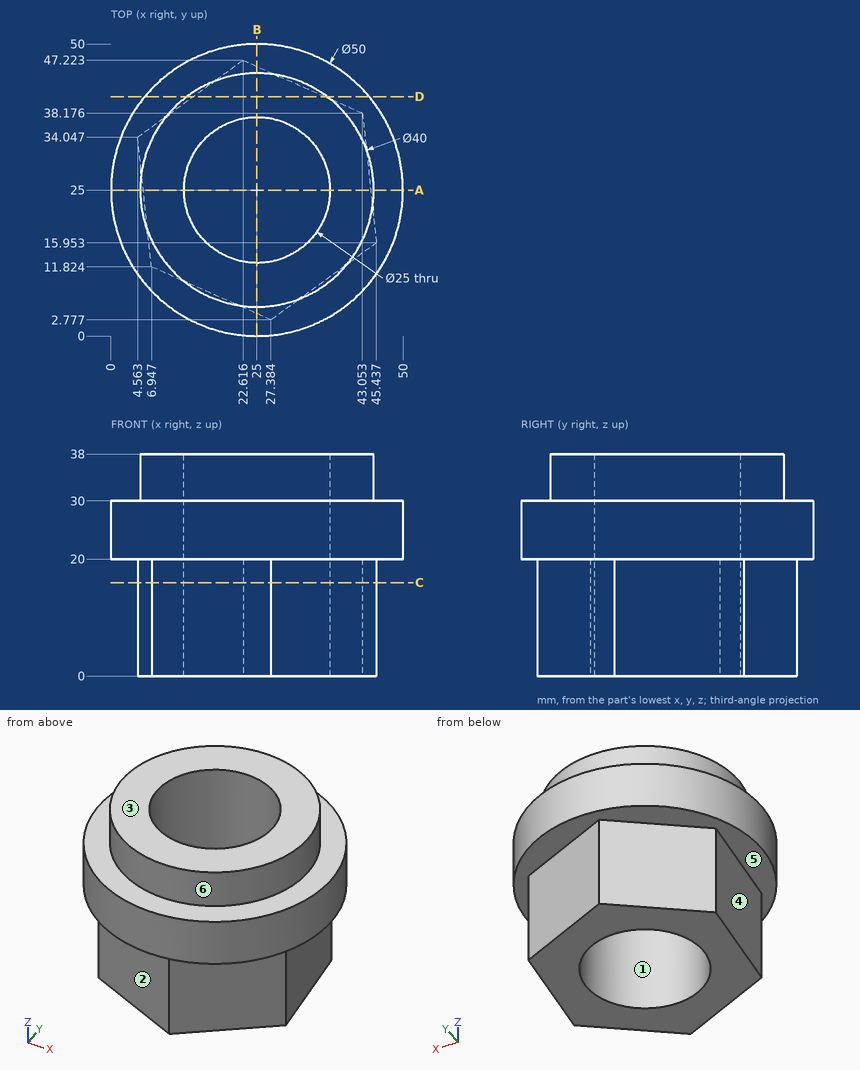
Job drawing, mm, ordinate dimensions from the low corner. One solid piece. A direction names the side the tool comes from. Coordinates: 2 decimals unless noted, no trailing zeros. Order: outer loops, then holes, each group sorted by start corner. A loop starts at its lowest first (then second) coordinate and runs counter-clockwise, first axis right, second up. Notation, with made-up numbers: M 80.25,82 L 129.25,82 A20 ccw 129.25,108 Z; hole C 88,-15.5 d6. An arc over 180 degrees is marked long. Return JSON: item names as keys, results as strings.
1. Pull direction X, two halves, no side cores. Call the marked faces 1, 2 and 3: +X half, -X half, draft (parallel to the pull), parting line (faces both ways), or undercut.
Ans:
{"face 1": "undercut", "face 2": "-X half", "face 3": "draft"}
2. Tool access for the marked faces 4, 5 and 6: list every direction of +Z, -Z, +X, -X, +Y, -Y with a clear straight run to the whole face (end or side of a thin tool).
Ans:
{"face 4": "-Z, -X, -Y", "face 5": "-Z", "face 6": "+Z"}
3. Saw through at A-A (y = 25). Give the cut face in (x, z).
Ans:
{"outline": "M 0,20 L 5.53,20 L 5.53,0 L 12.5,0 L 12.5,38 L 5,38 L 5,30 L 0,30 Z; M 37.5,0 L 44.47,0 L 44.47,20 L 50,20 L 50,30 L 45,30 L 45,38 L 37.5,38 Z"}
4. Saw through at B-B (x = 25). Give the cut face in (y, z).
Ans:
{"outline": "M 0,20 L 3.83,20 L 3.83,0 L 12.5,0 L 12.5,38 L 5,38 L 5,30 L 0,30 Z; M 37.5,0 L 46.17,0 L 46.17,20 L 50,20 L 50,30 L 45,30 L 45,38 L 37.5,38 Z"}
5. Flat gauge pins, fed straight in: pin 1 (10 mm diameter, centred on y = 11.5, z = 6.5, fed in from -X) (1 decimal); pin 2 (25 mm diameter, centred on x = 37, y = 18.5, fed in from -Z); pin 3 (5 mm diameter, centred on y = 34, z = 28.5, fed in from +X); pin 4 (2 mm diameter, centred on y = 11, z = 29, fed in from +X) (1 decimal). Where does each tip first touch, or does it go through?
Ans:
{"pin 1": "x = 6.4", "pin 2": "z = 0", "pin 3": "x = 49.14", "pin 4": "x = 46.4"}
6. Drill centre lines: probe 1 along Y at (x, z) = (25, 23.5); probe 2 along Y at (x, z) = (33.5, 25) (1 decimal); probe 3 along Z at (x, y) = (9.5, 42.5). Where is each one in solid material? Low to high.
Ans:
{"probe 1": "0 to 12.5, 37.5 to 50", "probe 2": "1.5 to 15.8, 34.2 to 48.5", "probe 3": "20 to 30"}
7. Saw through at D-D (y = 41). Give the cut face in (x, z), and give its area (3 significant figures).
Ans:
{"outline": "M 5.79,20 L 14.09,20 L 14.09,0 L 36.67,0 L 36.67,20 L 44.21,20 L 44.21,30 L 37,30 L 37,38 L 13,38 L 13,30 L 5.79,30 Z", "area": "1,030 mm^2"}
8. Saw through at C-C (z = 16). Give the cut face in (x, y) (1 decimal), and give its area (3 significant figures).
Ans:
{"outline": "M 4.6,34 L 6.9,11.8 L 27.4,2.8 L 45.4,16 L 43.1,38.2 L 22.6,47.2 Z; hole C 25,25 d25", "area": "807 mm^2"}
